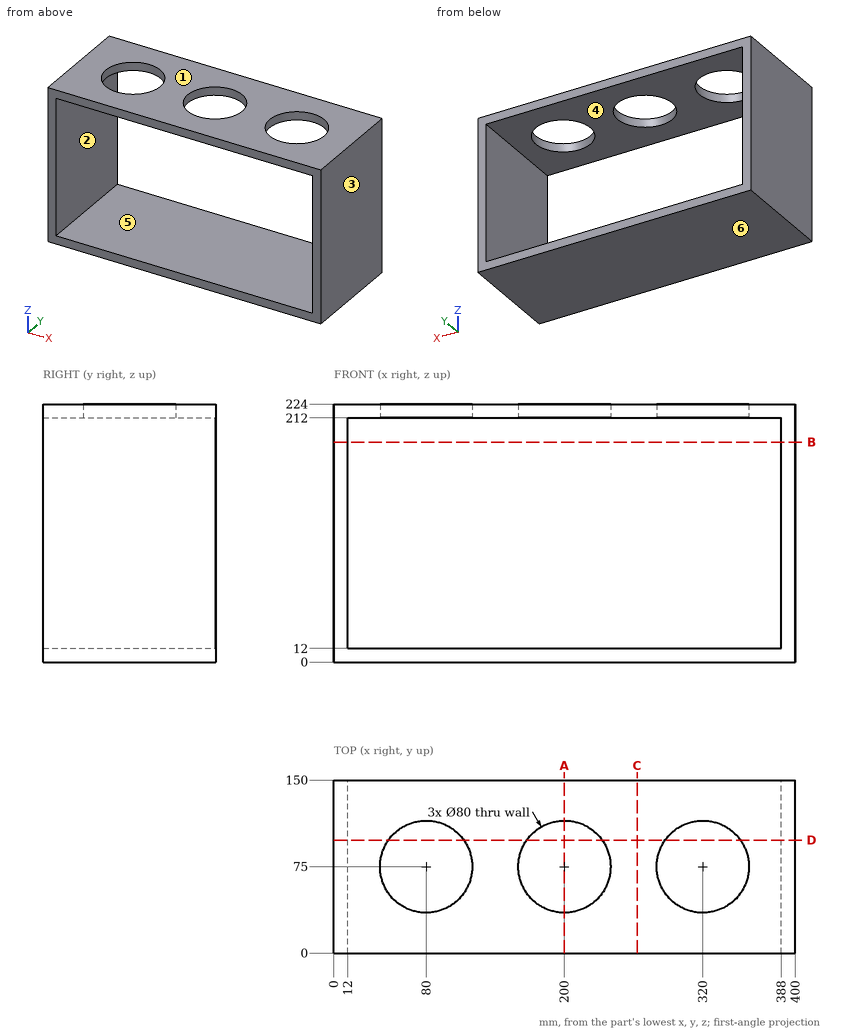
Study the drawing (mm; zero at the part's minimum x, y, z) and answer. A direction names the side the tool comes from. Coordinates: 2 decimals unless noted, no trailing zeros. Loops run counter-clockwise (first coordinate to the right, second up) from the corner with the lowest first, then second, coordinate; pieces in that order, holes last. Notation, with made-up numbers: M -1,66 L 30,66 A24 cw 30,80 Z; hole C 10.5,14.5 d6. An arc over 180 degrees is marked long. Answer in a Markdown table with one row per item.
1) Which of the six approach directions +Z, -Z, +X, -X, +Y, -Y give full straight-line access (tool end or side, diameter ignored) to the marked faces 5 and 6?
Answers below:
| item | result |
|---|---|
| face 5 | +Y, -Y |
| face 6 | -Z, +X, -X, +Y, -Y |
2) Find the intervals of material crossed by probe 1 along X at (y, z) = (114.5, 15.5); probe 2 along Z at (x, y) = (17, 35); probe 3 along Y at (x, z) = (80, 219.25), in increasing order.
Answers below:
| item | result |
|---|---|
| probe 1 | 0 to 12, 388 to 400 |
| probe 2 | 0 to 12, 212 to 224 |
| probe 3 | 0 to 35, 115 to 150 |
3) Find section D-D (y = 98). Determine the outline of the cut face in (x, z).
Answers below:
| item | result |
|---|---|
| outline | M 0,0 L 400,0 L 400,224 L 352.73,224 L 352.73,212 L 388,212 L 388,12 L 12,12 L 12,212 L 47.27,212 L 47.27,224 L 0,224 Z; M 112.73,212 L 167.27,212 L 167.27,224 L 112.73,224 Z; M 232.73,212 L 287.27,212 L 287.27,224 L 232.73,224 Z |
4) Find section C-C (x = 263). Determine the outline of the cut face in (y, z).
Answers below:
| item | result |
|---|---|
| outline | M 0,0 L 150,0 L 150,12 L 0,12 Z; M 0,212 L 150,212 L 150,224 L 0,224 Z |
5) Given pin 1 (3 mm diameter, centred on x = 84.5, y = 76.5, fed in from +Z), flat-ended and moving along its own axis, determine where the tip first touches the part or whether it passes through.
Answers below:
| item | result |
|---|---|
| pin 1 | z = 12 |
6) Determine the mould class of the marked faces 1, 2, 3 and 4 for opening direction Z: released by +Z, released by -Z, zero draft, split by the parting line, or undercut.
Answers below:
| item | result |
|---|---|
| face 1 | released by +Z |
| face 2 | undercut |
| face 3 | zero draft |
| face 4 | undercut |
7) Find section B-B (z = 191). Determine the outline of the cut face in (x, y).
Answers below:
| item | result |
|---|---|
| outline | M 0,0 L 12,0 L 12,150 L 0,150 Z; M 388,0 L 400,0 L 400,150 L 388,150 Z |
8) Find section A-A (x = 200). Determine the outline of the cut face in (y, z), then the cut area to 3 significant figures.
Answers below:
| item | result |
|---|---|
| outline | M 0,0 L 150,0 L 150,12 L 0,12 Z; M 0,212 L 35,212 L 35,224 L 0,224 Z; M 115,212 L 150,212 L 150,224 L 115,224 Z |
| area | 2,640 mm^2 |
